Can you work these out from the model? Positions are in its coordinate system, mm. Face numbers are marked on the shaded views. A direction names the side the tool comes from. Round coordinates to 2 decimals unless told otherwise and drop trailing zeros. Order: outer loops, then holes, each group sorted by start corner. A loop starts at its lowest first (then second) coordinate and runs counter-clockwise, first axis right, second up.
Q1. If we section it at C-C (z = 15.25): Please give me the cut outline in (x, y).
Q2. If we section it at A-A (x = 0): Please give me the cut outline in (y, z).
Q3. If I drill on line 1 (X direction, y = 3.25, z = 15.25); line 2 (Y direction, x = 0, z = 2.25); line 3 (Z direction, x = 3.45, y = 0), over which ranges is the centre line in solid material (lowest first)?
Q4. If we section it at B-B (z = 13): Please give me the cut outline in (x, y), plus the area to 3 significant figures.
Q5. We'd pull the mould along X, two halves only. Please class the marked faces 3, 4, 5 and 6: pulls with the +X half, pulls with the -X half, needs draft (parallel to the pull), parting line crosses it, or undercut.
Q6. If we section it at D-D (z = 4.75): Please give me the cut outline in (x, y), plus the area to 3 significant figures.
Q7. For the marked faces 1 and 2, which set-ups out of +Z, -Z, +X, -X, +Y, -Y let a thin tool reach every point of the face, with its end or its side?
Q8. Will these pins go through, and if not, where does the flat tip stop? P1, Ø3, axis at x = 0, y = 0, coming from the +Z side; P2, Ø5, axis at y = 0, z = 15.73, coming from the -X side; P3, Ø2, axis at y = -0.5, z = 17.5, coming from the +X side; P4, Ø2, axis at x = 0, y = 3.5, coming from the +Z side.
from build123d import *

# Parameters (mm, degrees)
SKETCH_1_R          = 6
SKETCH_1_R_2        = 2
EXTRUDE_1_DEPTH     = 10
EXTRUDE_2_DEPTH     = 10
SKETCH_3_R          = 2
CUT_EXTRUDE_3_DEPTH = 24.600847442
FILLET_1_R          = 1


with BuildPart() as part:
    # Эскиз1 → Вытянуть1 (new body)
    with BuildSketch(Plane.XY):
        Circle(SKETCH_1_R)
        Circle(SKETCH_1_R_2, mode=Mode.SUBTRACT)
    extrude(amount=EXTRUDE_1_DEPTH)

    # Эскиз2 → Вытянуть2 (add)
    with BuildSketch(Plane.XY.offset(10)):
        with BuildLine():
            Line((-5, 3.31662479), (-5, -3.31662479))
            ThreePointArc((-5, -3.31662479), (-3.69041576, -4.730838353), (-2, -5.656854249))
            Line((-2, -5.656854249), (-2, 5.656854249))
            ThreePointArc((-2, 5.656854249), (-3.69041576, 4.730838353), (-5, 3.31662479))
        make_face()
        with BuildLine():
            Line((2, 5.656854249), (2, -5.656854249))
            ThreePointArc((2, -5.656854249), (3.69041576, -4.730838353), (5, -3.31662479))
            Line((5, -3.31662479), (5, 3.31662479))
            ThreePointArc((5, 3.31662479), (3.69041576, 4.730838353), (2, 5.656854249))
        make_face()
    extrude(amount=EXTRUDE_2_DEPTH)

    # Эскиз3 → Вытянуть3 (cut, through all)
    with BuildSketch(Plane.ZY.offset(5)):
        with Locations(Location((15.728074635, 0, 0), (0, 0, 270))):
            Circle(SKETCH_3_R)
    extrude(amount=-CUT_EXTRUDE_3_DEPTH, mode=Mode.SUBTRACT)

    # Скругление1
    fillet_1_edges = [part.edges().sort_by_distance(p)[0] for p in [
        (-3.69041576, 4.730838353, 20),
        (-3.69041576, -4.730838353, 20),
        (3.69041576, -4.730838353, 20),
        (3.69041576, 4.730838353, 20),
    ]]
    fillet(fillet_1_edges, radius=FILLET_1_R - 0.0001)  # a hair under: the kernel refuses the full size


solid = part.part
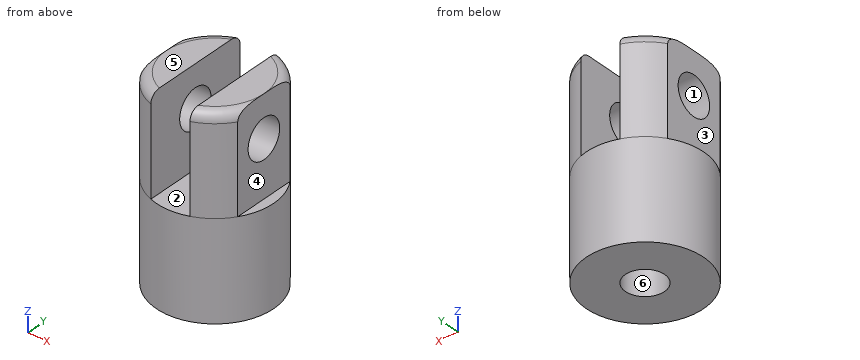
Solution:
1. outline: (-5, -3.32) arc R6 ccw to (-2, -5.66) - (-2, -1.94) - (-5, -1.94) - close; (-5, 1.94) - (-2, 1.94) - (-2, 5.66) arc R6 ccw to (-5, 3.32) - close; (2, -5.66) arc R6 ccw to (5, -3.32) - (5, -1.94) - (2, -1.94) - close; (2, 1.94) - (5, 1.94) - (5, 3.32) arc R6 ccw to (2, 5.66) - close
2. outline: (-6, 0) - (-2, 0) - (-2, 10) - (-6, 10) - close; (2, 0) - (6, 0) - (6, 10) - (2, 10) - close
3. line 1: x = -5 to -2, 2 to 5
3. line 2: y = -6 to -2, 2 to 6
3. line 3: z = 0 to 13.73, 17.73 to 20
4. outline: (-5, -3.32) arc R6 ccw to (-2, -5.66) - (-2, 5.66) arc R6 ccw to (-5, 3.32) - close; (2, -5.66) arc R6 ccw to (5, -3.32) - (5, 3.32) arc R6 ccw to (2, 5.66) - close
4. area: 57.0 mm2
5. face 3: pulls with the -X half
5. face 4: pulls with the +X half
5. face 5: needs draft
5. face 6: undercut
6. outline: circle Ø12 at (0, 0); hole circle Ø4 at (0, 0)
6. area: 101 mm2
7. face 1: +X, -X
7. face 2: +Z, +Y, -Y
8. P1: passes through
8. P2: stops at x = -5
8. P3: stops at x = 5
8. P4: stops at z = 10
